Geometry check sheet. Reference: the model listing, model coordinates, mm. Coordinates: 2 decimals unless noted, no trailing zeros. Loops run counter-clockwise (first coordinate to the right, second up) from the corner with the lowest first, then second, coordinate; pieces in that order, holes last. Notation, with made-up numbers: (11.5, 37.25) - (65.5, 37.25) arc R23 ccw to (65.5, 66.25) - close; hole circle Ø8 at (-36, -18.5). An arc over 180 degrees is marked (long way). Write item = value, one per line. Start each with the question number.
from build123d import *

# Parameters (mm, degrees)
BOSS_EXTRUDE1_DEPTH                          = 1.5
CSK_FOR_M3_COUNTERSUNK_FLAT_HEAD_SCR_2_COUNT = 2
CSK_FOR_M3_COUNTERSUNK_FLAT_HEAD_SCR_2_PITCH = 8


with BuildPart() as part:
    # Sketch1 → Boss-Extrude1 (new, symmetric)
    with BuildSketch(Plane(origin=(0, 0, 0), x_dir=(0, 0, -1), z_dir=(1, 0, 0))):
        with BuildLine():
            Line((5, 5), (5, -5))
            ThreePointArc((5, -5), (0, -10), (-5, -5))
            Line((-5, -5), (-5, 5))
            ThreePointArc((-5, 5), (0, 10), (5, 5))
        make_face()
    extrude(amount=BOSS_EXTRUDE1_DEPTH, both=True)

    # Sketch3 → CSK for M3 Countersunk Flat Head Screw1 (revolve, cut)
    with BuildSketch(Plane(origin=(1.5, 4, 0), x_dir=(0, 0, -1), z_dir=(0, 1, 0))):
        Polygon((0, 0), (0, 3), (1.7, 3), (1.7, 1.45), (3.15, 0), align=None)
    csk_for_m3_countersunk_flat_head_screw1 = revolve(axis=Axis((7.85, 4, 0), (-1, 0, 0)), mode=Mode.SUBTRACT)

    # CSK for M3 Countersunk Flat Head Scr 2: CSK for M3 Countersunk Flat Head Screw1 ×2
    with Locations(*[(0, -i * CSK_FOR_M3_COUNTERSUNK_FLAT_HEAD_SCR_2_PITCH, 0) for i in range(1, CSK_FOR_M3_COUNTERSUNK_FLAT_HEAD_SCR_2_COUNT)]):
        add(csk_for_m3_countersunk_flat_head_screw1, mode=Mode.SUBTRACT)


solid = part.part
(1) Sectioned sample at B-B on y = 4. Enter the section's corners in (x, z).
(2) Sectioned sample at C-C on x = -0.55. Enter the section's corners in (y, z), plus the area to 3 significant figures.
(3) Draft check along Z on faces 1 (the face through (-0.71, -2.34, 0.37)), 2 (the face through (0, 0, -5)), 3 (the face through (0, 10, 0)). Enter one of: pulls with the +Z half, pulls with the -Z half, needs draft (parallel to the pull), parting line crosses it, or undercut.
(4) Sectioned sample at D-D on x = 1. Enter the section's corners in (y, z).
(5) Scan lines: line 1 (Y direction, x = -0.6, z = 0); line 2 (Z direction, x = -0.6, y = -4); line 3 (Y direction, x = -1.2, z = 1.5). Record each from-to range of solid material in increasing order.
(6) Depth check by flat-ended pin: pin 1 (4 mm diameter, centred on y = -4, z = 0, fed in from +X); pin 2 (4.5 mm diameter, centred on y = 4, z = 0, fed in from +X). Enter the tip coordinate at first touch or a pass-through.
(7) Sectioned sample at A-A on z = 0. Enter the section's corners in (x, y), plus the area to 3 significant figures.
Working result:
q1.outline = (-1.5, -5) - (1.5, -5) - (1.5, -3.15) - (0.05, -1.7) - (-1.5, -1.7) - close; (-1.5, 1.7) - (0.05, 1.7) - (1.5, 3.15) - (1.5, 5) - (-1.5, 5) - close
q2.outline = (-5, -5) - (5, -5) arc R5 ccw to (5, 5) - (-5, 5) arc R5 ccw to start; hole circle Ø3.4 at (-4, 0); hole circle Ø3.4 at (4, 0)
q2.area = 160 mm2
q3.face_1 = undercut
q3.face_2 = pulls with the -Z half
q3.face_3 = parting line crosses it
q4.outline = (-5, -5) - (5, -5) arc R5 ccw to (5, 5) - (-5, 5) arc R5 ccw to start; hole circle Ø5.3 at (-4, 0); hole circle Ø5.3 at (4, 0)
q5.line_1 = -10 to -5.7, -2.3 to 2.3, 5.7 to 10
q5.line_2 = -5 to -1.7, 1.7 to 5
q5.line_3 = -9.77 to -4.8, -3.2 to 3.2, 4.8 to 9.77
q6.pin_1 = 0.35
q6.pin_2 = 0.6
q7.outline = (-1.5, -10) - (1.5, -10) - (1.5, -7.15) - (0.05, -5.7) - (-1.5, -5.7) - close; (-1.5, -2.3) - (0.05, -2.3) - (1.5, -0.85) - (1.5, 0.85) - (0.05, 2.3) - (-1.5, 2.3) - close; (-1.5, 5.7) - (0.05, 5.7) - (1.5, 7.15) - (1.5, 10) - (-1.5, 10) - close
q7.area = 35.4 mm2
